For this review, use the dimensioned drawing (mm, ordinates from the lowest corner) and the shaded views. A direction names the side the tool comes from. Coordinates: 2 decimals unless noted, no trailing zeros. Order: outer loops, then holes, each group sorted by start corner. A loop starts at its lowest first (then second) coordinate and runs counter-clockwise, first axis right, second up. Notation, with made-up numbers: M -10.5,46 L 46.5,46 A31 cw 46.5,70 Z; hole C 23,79.25 d8. An arc over 180 degrees is marked long. Answer in a Markdown table with one row per item.
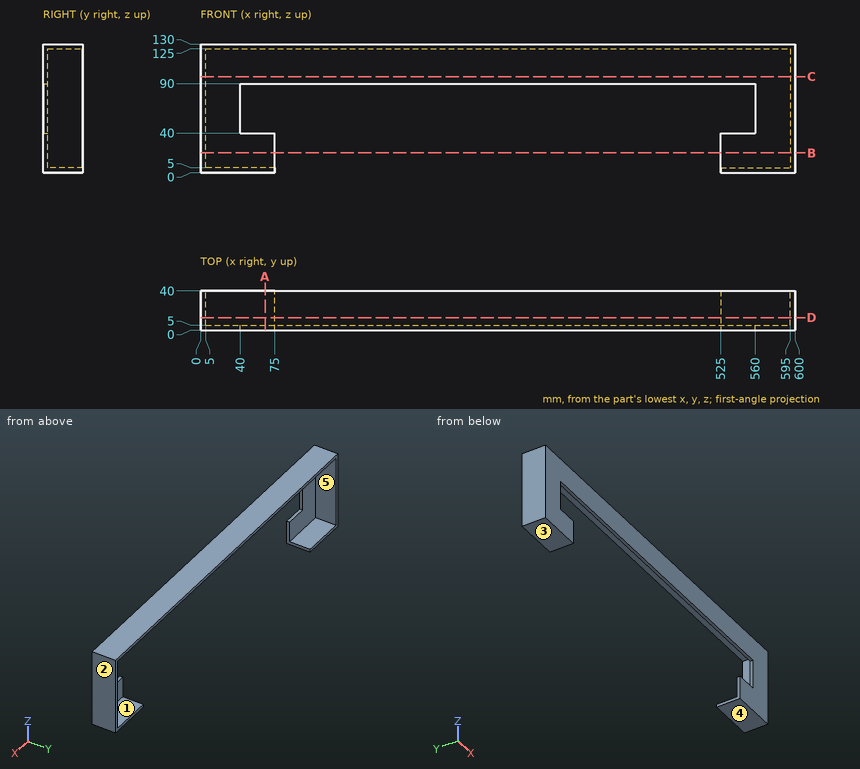
(1) Add section C-C, the plane z = 97. Give the boundary of the cut face in (x, y).
Return value:
| item | result |
|---|---|
| outline | M 0,0 L 600,0 L 600,40 L 595,40 L 595,5 L 5,5 L 5,40 L 0,40 Z |
(2) For line 1 along X through (y, z) = (11.5, 107.5); line 2 along Z through (x, y) = (557.5, 24); line 3 along Z through (x, y) = (335.5, 6), list the stretches that pass through material, from the lowest coordinate up. Write a range as from..to.
Return value:
| item | result |
|---|---|
| line 1 | x = 0..5, 595..600 |
| line 2 | z = 0..5, 125..130 |
| line 3 | z = 125..130 |
(3) Add section A-A, the plane x = 65. Give the boundary of the cut face in (y, z), and give its area (3 significant figures).
Return value:
| item | result |
|---|---|
| outline | M 0,0 L 40,0 L 40,5 L 5,5 L 5,40 L 0,40 Z; M 0,90 L 5,90 L 5,125 L 40,125 L 40,130 L 0,130 Z |
| area | 750 mm2 |
(4) Add section D-D, the plane y = 13. Give the boundary of the cut face in (x, z), and give its area (3 significant figures).
Return value:
| item | result |
|---|---|
| outline | M 0,0 L 75,0 L 75,5 L 5,5 L 5,125 L 595,125 L 595,5 L 525,5 L 525,0 L 600,0 L 600,130 L 0,130 Z |
| area | 4,950 mm2 |
(5) Draft analysis for pull direction Z (two halves, no side actions). For the marked faces 1, 2 and 3, state which applies: pulls with the +Z half, pulls with the -Z half, needs draft (parallel to the pull), parting line crosses it, or undercut.
Return value:
| item | result |
|---|---|
| face 1 | undercut |
| face 2 | needs draft |
| face 3 | pulls with the -Z half |
(6) Insertion check: pin 1 Ø10.5 at (x, y) = (272.5, 16.5) entering from -Z; pin 2 Ø3 at (x, z) = (534.5, 91) entering from +Y; pin 3 Ø4 at (x, y) = (252, 2.5) entering from -Z. Each pin has a flat end and moves straight along its axis. Give the tip position at first contact, or say it passes through.
Return value:
| item | result |
|---|---|
| pin 1 | stops at z = 125 |
| pin 2 | stops at y = 5 |
| pin 3 | stops at z = 90 |
(7) For the marked faces 4 and 5, list the 3-axis set-ups (+Z, -Z, +X, -X, +Y, -Y) from which the entire face can be reached by the end or side of a thin tool; tool diameter is ignored.
Return value:
| item | result |
|---|---|
| face 4 | -Z, +X, -X, +Y, -Y |
| face 5 | +Y |
(8) Add section B-B, the plane z = 20. Give the boundary of the cut face in (x, y).
Return value:
| item | result |
|---|---|
| outline | M 0,0 L 75,0 L 75,5 L 5,5 L 5,40 L 0,40 Z; M 525,0 L 600,0 L 600,40 L 595,40 L 595,5 L 525,5 Z |
